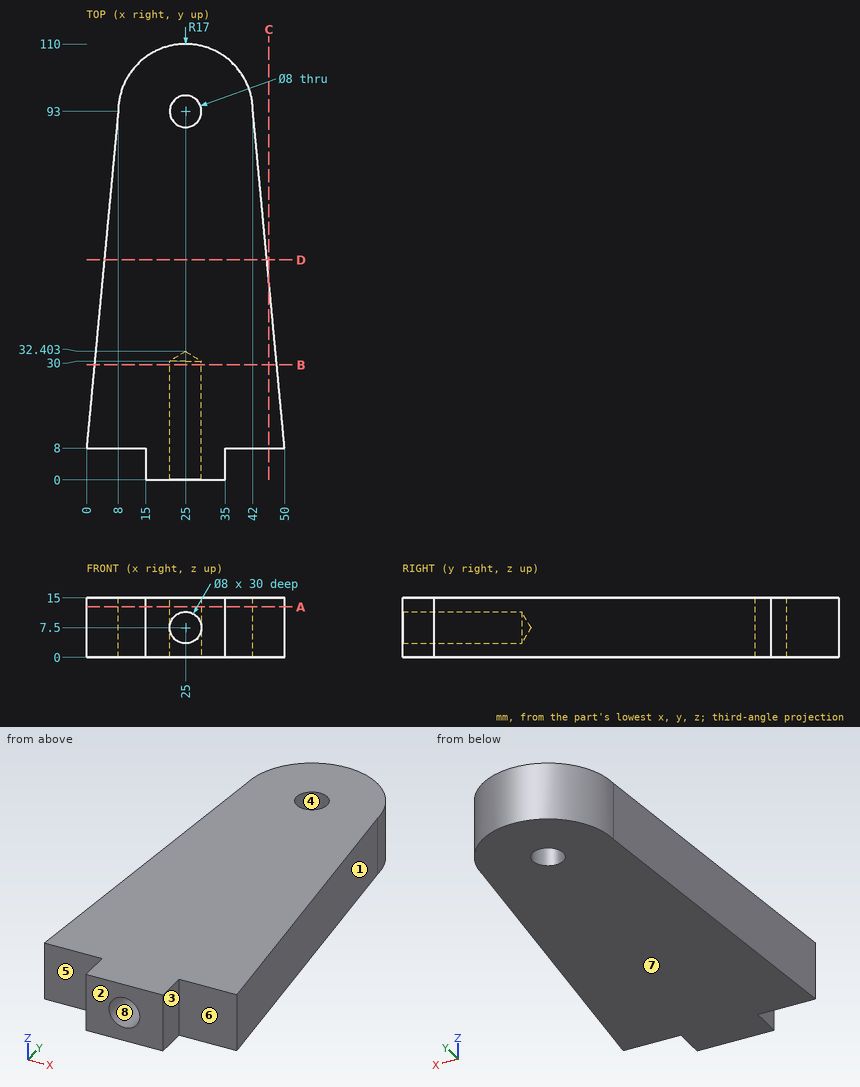
The figure shows three views and two pictorial views of one solid part (mm, origin at its lowest corner). Answer the questions. A direction names the side the tool comes from. Give positions to 0.01 mm unless a question says otherwise; leave off trailing zeros. Order: outer loops, then holes, each group sorted by start corner. A loop starts at its lowest first (then second) coordinate and runs counter-clockwise, first axis right, second up. Notation, with made-up numbers: (14, 3.5) -> (61, 3.5) arc R6 cw to (61, 12.5) -> close; hole circle Ø10 at (28, -18.75). An arc over 180 degrees is marked (long way). One line per item, written item: value.
1) Determine the mould class of the marked faces 1, 2, 3 and 4 for opening direction Y: pulls with the +Y half, pulls with the -Y half, needs draft (parallel to the pull), parting line crosses it, or undercut.
Reported:
face 1: pulls with the +Y half
face 2: pulls with the -Y half
face 3: needs draft
face 4: undercut
2) Find section A-A, the plane z = 12.75. Determine the outline of the cut face in (x, y), plus the area to 3 significant figures.
Reported:
outline: (0, 8) -> (15, 8) -> (15, 0) -> (35, 0) -> (35, 8) -> (50, 8) -> (42, 93) arc R17 ccw to (8, 93) -> close; hole circle Ø8 at (25, 93)
area: 4,130 mm^2
3) A tool of negligible diameter and unlimited length cuts with its end or side. For the marked faces 5, 6, 7 and 8, from which of +Z, -Z, +X, -X, +Y, -Y can it reach the whole face along a straight path? Write none if from no direction.
Reported:
face 5: +Z, -Z, -X, -Y
face 6: +Z, -Z, +X, -Y
face 7: -Z, +X, -X, +Y, -Y
face 8: -Y
4) Find section C-C, the plane x = 46. Determine the outline of the cut face in (y, z).
Reported:
outline: (8, 0) -> (50.5, 0) -> (50.5, 15) -> (8, 15) -> close
5) Find section D-D, the plane y = 55.5. Determine the outline of the cut face in (x, z), plus the area to 3 significant figures.
Reported:
outline: (4.47, 0) -> (45.53, 0) -> (45.53, 15) -> (4.47, 15) -> close
area: 616 mm^2
6) Find section B-B, the plane y = 29. Determine the outline of the cut face in (x, z).
Reported:
outline: (1.98, 0) -> (48.02, 0) -> (48.02, 15) -> (1.98, 15) -> close; hole circle Ø8 at (25, 7.5)
7) Flat-ended cylindrical pins translate along their axes: P1, Ø9, axis at y = 2.5, z = 9.5, coming from the -X side; P2, Ø2.5, axis at y = 6, z = 7, coming from the +X side; P3, Ø8, axis at y = 18, z = 2.5, coming from the +X side (1 decimal). Find the tip coordinate at first contact, or state that the pin passes through.
Reported:
P1: stops at x = 15
P2: stops at x = 35
P3: stops at x = 49.4
8) Find the intervals of material crossed by line 1 (Z direction, x = 25, y = 16.5); line 2 (Y direction, x = 25, z = 7.5) (1 decimal); line 3 (Y direction, x = 25, z = 3.25), in increasing order.
Reported:
line 1: z = 0 to 3.5, 11.5 to 15
line 2: y = 32.4 to 89, 97 to 110
line 3: y = 0 to 89, 97 to 110
